The listing builds one solid part. Answer for the finished solid, in the listing's coordinates (mm). A direction names the side the tool comes from. Give positions to 0.01 mm unless a question says otherwise; leave off trailing zeros. Order: outer loops, then holes, each group sorted by start corner. A loop starts at its lowest first (then second) coordinate and runs counter-clockwise, first axis right, second up. Notation, with made-up numbers: (-26.75, 34.25) -> (12.25, 34.25) arc R24 cw to (12.25, 64.25) -> close; hole circle Ø10 at (-23, 30.25). An arc over 180 degrees is marked (long way). One line per question, with ' | ' between items. Start each with the question number.
```python
from build123d import *

# Parameters (mm, degrees)
F1_DEPTH = 25.4
F3_DEPTH = 25.401
F4_R     = 6.353022
F5_DEPTH = 25.401
F8_DEPTH = 25.4
F9_DEPTH = 25.4


with BuildPart() as f1:
    # F0 (on Front) → F1 (new body)
    with BuildSketch(Plane.XZ):
        Polygon((-20.024838, 38.1), (-45.424838, 38.1), (-45.424838, 0), (24.425162, 0), (24.827223, 12.7), (-20.024838, 12.7), align=None)
    extrude(amount=F1_DEPTH)

    # F2 (on face) → F3 (cut, through all)
    with BuildSketch(Plane.XZ.offset(25.4)):
        with BuildLine():
            ThreePointArc((-45.424838, 25.4), (-32.724838, 37.822931), (-20.024838, 25.4))
            Line((-20.024838, 25.4), (-20.024838, 38.1))
            Line((-20.024838, 38.1), (-45.424838, 38.1))
            Line((-45.424838, 38.1), (-45.424838, 25.4))
        make_face()
    extrude(amount=-F3_DEPTH, mode=Mode.SUBTRACT)

    # F4 (on face) → F5 (cut, through all)
    with BuildSketch(Plane.XZ.offset(25.4)):
        with Locations((-32.724838, 25.122931)):
            Circle(F4_R)
    extrude(amount=-F5_DEPTH, mode=Mode.SUBTRACT)

    # F7 (on face) → F8 (cut)
    with BuildSketch(Plane.XY.offset(12.7)):
        with BuildLine():
            ThreePointArc((-7.324838, -19.203114), (-2.834065, -17.342975), (-0.973926, -12.852202))
            ThreePointArc((-0.973926, -12.852202), (-2.834065, -8.361429), (-7.324838, -6.50129))
            ThreePointArc((-7.324838, -6.50129), (-13.67575, -12.852202), (-7.324838, -19.203114))
        make_face()
        with BuildLine():
            ThreePointArc((-7.324838, -6.50129), (-2.834065, -8.361429), (-0.973926, -12.852202))
            ThreePointArc((-0.973926, -12.852202), (-2.834065, -17.342975), (-7.324838, -19.203114))
            Line((-7.324838, -19.203114), (12.127223, -19.200703))
            ThreePointArc((12.127223, -19.200703), (5.77634, -12.849819), (12.127223, -6.498936))
            Line((12.127223, -6.498936), (-7.324838, -6.50129))
        make_face()
        with BuildLine():
            ThreePointArc((18.478107, -12.849819), (16.617976, -8.359066), (12.127223, -6.498936))
            ThreePointArc((12.127223, -6.498936), (5.77634, -12.849819), (12.127223, -19.200703))
            ThreePointArc((12.127223, -19.200703), (16.617976, -17.340572), (18.478107, -12.849819))
        make_face()
    extrude(amount=-F8_DEPTH, mode=Mode.SUBTRACT)

    # F7 (on face) → F9 (cut)
    with BuildSketch(Plane.XY.offset(12.7)):
        with BuildLine():
            ThreePointArc((19.19838, 0), (24.668979, -12.534609), (20.029411, -25.4))
            Line((20.029411, -25.4), (24.827223, -25.4))
            Line((24.827223, -25.4), (24.827223, 0))
            Line((24.827223, 0), (19.19838, 0))
        make_face()
    extrude(amount=-F9_DEPTH, mode=Mode.SUBTRACT)


solid = f1.part
```
(1) The part is cut by section B-B on x = 3. Determine the outline of the cut face in (y, z), plus the area to 3 significant figures.
(2) The part is cut by section D-D on z = 28.5. Determine the outline of the cut face in (x, y), plus the area to 3 significant figures.
(3) Given P1, Ø3, axis at x = -5.5, z = 14.5, coming from the +Y side; P2, Ø8, axis at y = -3.5, z = 31, coming from the -X side; P3, Ø4, axis at y = -10.5, z = 18, coming from the +X side; P4, Ø6, axis at y = -16.5, z = 15, coming from the +X side, each flat-ended and moving along its own axis, determine where each tip first touches the part or whether it passes through.
(4) The part is cut by section C-C on z = 10. Determine the outline of the cut face in (x, y), plus the area to 3 significant figures.
(5) Determine the mould class of faces 1 (the face through (-45.425, -13, 13)), 2 (the face through (3, -21, 12.7)), 3 (the face through (-34.1, -12.88, 18.92)) for opening direction Z: pulls with the +Z half, pulls with the -Z half, needs draft (parallel to the pull), parting line crosses it, or undercut.
(6) For faces 4 (the face through (-20.4, -25.4, 15)), 5 (the face through (-20.025, -13, 19)), 6 (the face through (-13.674, -12.713, 6.439)), determine the directions among +Z, -Z, +X, -X, +Y, -Y from which every point of the face is accessible in a straight line to the end or side of a thin tool.
(7) Consider line 1 (X direction, y = -20, z = 25); line 2 (Y direction, x = 8, z = 11); line 3 (X direction, y = -7, z = 17). Determine where each line is inside the solid, lowest interval first.
Result sheet:
1) outline: (-25.4, 0) -> (-19.2, 0) -> (-19.2, 12.7) -> (-25.4, 12.7) -> close; (-6.5, 0) -> (0, 0) -> (0, 12.7) -> (-6.5, 12.7) -> close | area: 161 mm^2
2) outline: (-44.97, -25.4) -> (-38.11, -25.4) -> (-38.11, 0) -> (-44.97, 0) -> close; (-27.34, -25.4) -> (-20.48, -25.4) -> (-20.48, 0) -> (-27.34, 0) -> close | area: 349 mm^2
3) P1: passes through | P2: stops at x = -45.29 | P3: stops at x = -20.02 | P4: stops at x = 24.62
4) outline: (-45.42, -25.4) -> (20.03, -25.4) arc R18.49 ccw to (19.2, 0) -> (-45.42, 0) -> close; hole (-7.32, -19.2) -> (12.13, -19.2) arc R6.35 ccw to (18.48, -12.85) arc R6.35 ccw to (12.13, -6.5) -> (-7.32, -6.5) arc R6.35 ccw to start | area: 1,370 mm^2
5) face 1: needs draft | face 2: pulls with the +Z half | face 3: undercut
6) face 4: +Z, -Z, +X, -X, -Y | face 5: +Z, +X, +Y, -Y | face 6: +Z, -Z
7) line 1: x = -45.42 to -39.08, -26.37 to -20.02 | line 2: y = -25.4 to -19.2, -6.5 to 0 | line 3: x = -45.42 to -20.02
